Work out the finished part from the listing and answer in its coordinate system (mm). Coordinates: 2 decimals unless noted, no trailing zeros. Order: outer loops, then holes, each group sorted by start corner. A loop starts at its lowest first (then second) coordinate and runs counter-clockwise, first axis right, second up.
1. The part is cut by section B-B, the plane z = 152. Give the vertices of the cut face in (x, y).
2. The part is cut by section A-A, the plane y = 6.5. Give the vertices of the cut face in (x, z).
3. Flat-ended cylindrical pins translate along their axes: pin 1 Ø1 at (x, y) = (4.5, 7.5) entering from -Z; pin 2 Ø4 at (x, y) = (-8, 2) entering from +Z; pin 3 Ø3 at (y, z) = (3, 115.5) entering from +X; pin 4 Ø10 at (x, z) = (3, 37) entering from +Y. Find the tip coordinate at first contact, or state that the pin passes through.
4. Find the intervals of material crossed by probe 1 along X at (y, z) = (3.25, 57); probe 2 along Z at (x, y) = (4.5, 1.75); probe 3 along Z at (x, y) = (-7, 4.5), in increasing order.
```python
from build123d import *

# Parameters (mm, degrees)
SKETCH1_W           = 9.5
SKETCH1_H           = 180
BOSS_EXTRUDE1_DEPTH = 10
FILLET1_R           = 1.9
FILLET2_R           = 4.75


with BuildPart() as part:
    # Sketch1 → Boss-Extrude1 (new body)
    with BuildSketch(Plane(origin=(0, 0, 0), x_dir=(1, 0, 0), z_dir=(0, 1, 0))):
        with Locations((-2.027493606, -84.590792839)):
            Rectangle(SKETCH1_W, SKETCH1_H)
        Polygon((-6.777493606, 5.409207161), (-2.027493606, 5.409207161), (-2.027493606, 14.909207161), (-16.277493606, 5.409207161), align=None)
        Polygon((-2.027493606, 14.909207161), (-2.027493606, 5.409207161), (2.722506394, 5.409207161), (12.222506394, 5.409207161), align=None)
        Polygon((-6.777493606, -174.590792839), (2.722506394, -174.590792839), (12.222506394, -174.590792839), (-1.277493606, -184.090792839), (-16.277493606, -174.590792839), align=None)
    extrude(amount=BOSS_EXTRUDE1_DEPTH)

    # Fillet1
    fillet1_edges = [part.edges().sort_by_distance(p)[0] for p in [
        (12.222506394, 5, -5.409207161),
        (12.222506394, 5, 174.590792839),
        (-16.277493606, 5, 174.590792839),
        (-16.277493606, 5, -5.409207161),
    ]]
    fillet(fillet1_edges, radius=FILLET1_R)

    # Fillet2
    fillet2_edges = [part.edges().sort_by_distance(p)[0] for p in [
        (-1.277493606, 5, 184.090792839),
        (-2.027493606, 5, -14.909207161),
    ]]
    fillet(fillet2_edges, radius=FILLET2_R)


solid = part.part
```
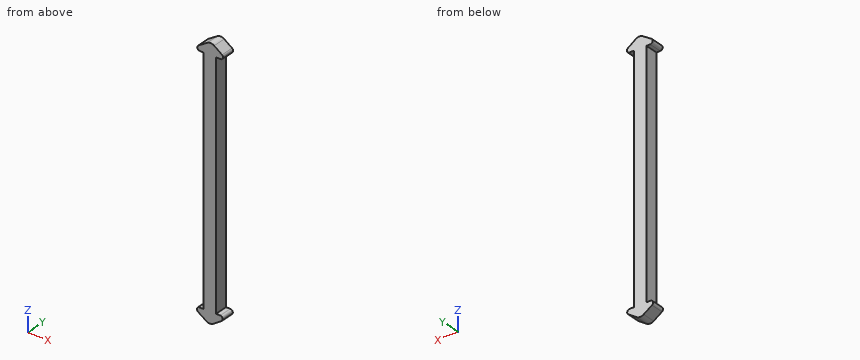
Geometry says:
1. outline: (-6.78, 0) - (2.72, 0) - (2.72, 10) - (-6.78, 10) - close
2. outline: (-11.06, -8.89) - (-4.66, -13.15) arc R4.75 ccw to (0.61, -13.15) - (7, -8.89) arc R1.9 ccw to (5.95, -5.41) - (2.72, -5.41) - (2.72, 174.59) - (6.22, 174.59) arc R1.9 ccw to (7.31, 178.04) - (1.32, 182.26) arc R4.75 ccw to (-3.96, 182.39) - (-10.74, 178.1) arc R1.9 ccw to (-9.73, 174.59) - (-6.78, 174.59) - (-6.78, -5.41) - (-10, -5.41) arc R1.9 ccw to start
3. pin 1: stops at z = -10.89
3. pin 2: stops at z = 181.1
3. pin 3: stops at x = 2.72
3. pin 4: stops at y = 10
4. probe 1: x = -6.78 to 2.72
4. probe 2: z = -10.56 to -5.41, 174.59 to 180.03
4. probe 3: z = -11.59 to -5.41, 174.59 to 180.47
